The model under review builds one solid part; all positions refer to its coordinate system, in mm. A direction names the side the tool comes from. Round coordinates to 2 decimals unless told otherwise and drop trailing zeros. Order: outer loops, then holes, each group sorted by start corner. A loop starts at its lowest first (then second) coordinate and runs counter-clockwise, first axis right, second up. Notation, with made-up numbers: (8.25, 76.5) - (45.25, 76.5) arc R16 cw to (45.25, 95.5) - close; hole circle Ø1 at (-18.5, 79.5). An arc over 180 degrees is marked (long way). One line per question, with ' | ' between items. Start each with the question number.
Item 1: Add section B-B on x = 1. State the section outline as (y, z) points, and give its area (3 significant figures).
Item 2: Add section D-D on z = -12.5. State the section outline as (x, y) points.
Item 3: Insertion check: pin 1 Ø1 at (y, z) = (-30, 18.5) entering from +X; pin 2 Ø10 at (y, z) = (-12.5, -15.5) entering from +X; pin 3 Ø3 at (x, z) = (26, 17.32) entering from +Y; pin 4 Ø7.5 at (y, z) = (6.5, 4) entering from -X. Each pin has a flat end and moves straight along its axis. Give the tip position at first contact, or say it passes through.
Item 4: Tool access review of faces 1 (the face through (1, 0, 0)), 2 (the face through (-30, 6, -6)), 3 (the face through (27.476, -51.521, -18.261)), 4 (the face through (9, 6, 22)), 5 (the face through (-18, 7, -21)): name each direction out of +Z, -Z, +X, -X, +Y, -Y from which nothing blocks a thin tool from reaching the whole face with its end or side.
Item 5: For L1, parallel to X at y = -51, z = 0; L2, parallel to Y at x = -24, z = 4.5; L3, parallel to Z at x = -15, y = -23.5, list the stretches that pass through material, from the lowest coordinate up. Write a range as [from, to].
Item 6: Add section A-A on y = 6. State the section outline as (x, z) points, and give its area (3 significant figures).
Item 7: Draft analysis for pull direction X (two halves, no side actions). For faces 6 (the face through (-31, -21, 0)), 7 (the face through (-30, 6, 6)), 8 (the face through (-7, 6, -22)), state which applies: +X half, -X half, draft (parallel to the pull), parting line (faces both ways), or undercut.
Item 8: Add section C-C on x = -13.5. State the section outline as (y, z) points.
from build123d import *

# Parameters (mm, degrees)
SKETCH_1_W          = 62
SKETCH_1_H          = 46
EXTRUDE_1_DEPTH     = 10
SKETCH_2_W          = 58
SKETCH_2_H          = 42
CUT_EXTRUDE_1_DEPTH = 7
CUT_EXTRUDE_2_REACH = 68.88
SKETCH_3_W          = 12
SKETCH_3_H          = 14
CUT_EXTRUDE_3_REACH = 56.745
SKETCH_5_W          = 36
SKETCH_5_H          = 7
CUT_EXTRUDE_4_REACH = 56.745
SKETCH_6_W          = 20
SKETCH_6_H          = 7
EXTRUDE_2_DEPTH     = 50
SKETCH_9_W          = 62
SKETCH_9_H          = 46
EXTRUDE_3_DEPTH     = 3
CUT_EXTRUDE_5_REACH = 75.885
SKETCH_10_R         = 1.75


with BuildPart() as part:
    # 草图1 → 凸台-拉伸1 (new body)
    with BuildSketch(Plane(origin=(0, 0, 0), x_dir=(1, 0, 0), z_dir=(0, 1, 0))):
        Rectangle(SKETCH_1_W, SKETCH_1_H)
    extrude(amount=EXTRUDE_1_DEPTH)

    # 草图2 → 切除-拉伸1 (cut)
    with BuildSketch(Plane(origin=(0, 10, 0), x_dir=(1, 0, 0), z_dir=(0, 1, 0))):
        Rectangle(SKETCH_2_W, SKETCH_2_H)
    extrude(amount=-CUT_EXTRUDE_1_DEPTH, mode=Mode.SUBTRACT)

    # 草图3 → 切除-拉伸2 (cut, up to next)
    with BuildSketch(Plane.ZY.offset(31), mode=Mode.PRIVATE) as cut_extrude_2_sk1:
        with Locations((0, 10)):
            Rectangle(SKETCH_3_W, SKETCH_3_H)
    cut_extrude_2_tool1 = extrude(cut_extrude_2_sk1.sketch, amount=-CUT_EXTRUDE_2_REACH, mode=Mode.PRIVATE) & part.part
    add(cut_extrude_2_tool1.solids().sort_by_distance((-31, 10, 0))[0], mode=Mode.SUBTRACT)

    # 草图5 → 切除-拉伸3 (cut, up to next)
    with BuildSketch(Plane.XY.offset(-21), mode=Mode.PRIVATE) as cut_extrude_3_sk1:
        with Locations((11, 6.5)):
            Rectangle(SKETCH_5_W, SKETCH_5_H)
    cut_extrude_3_tool1 = extrude(cut_extrude_3_sk1.sketch, amount=-CUT_EXTRUDE_3_REACH, mode=Mode.PRIVATE) & part.part
    add(cut_extrude_3_tool1.solids().sort_by_distance((11, 6.5, -21))[0], mode=Mode.SUBTRACT)

    # 草图6 → 切除-拉伸4 (cut, up to next)
    with BuildSketch(Plane(origin=(0, 0, 21), x_dir=(-1, 0, 0), z_dir=(0, 0, -1)), mode=Mode.PRIVATE) as cut_extrude_4_sk1:
        with Locations((-19, 6.5)):
            Rectangle(SKETCH_6_W, SKETCH_6_H)
    cut_extrude_4_tool1 = extrude(cut_extrude_4_sk1.sketch, amount=-CUT_EXTRUDE_4_REACH, mode=Mode.PRIVATE) & part.part
    add(cut_extrude_4_tool1.solids().sort_by_distance((19, 6.5, 21))[0], mode=Mode.SUBTRACT)

    # 草图8 → 凸台-拉伸2 (add)
    with BuildSketch(Plane.XZ):
        Polygon((0, -23), (0, -20), (-28, -20), (-28, 20), (0, 20), (0, 23), (-31, 23), (-31, -23), align=None)
    extrude(amount=EXTRUDE_2_DEPTH)

    # 草图9 → 凸台-拉伸3 (add)
    with BuildSketch(Plane.XZ.offset(50)):
        Rectangle(SKETCH_9_W, SKETCH_9_H)
    extrude(amount=EXTRUDE_3_DEPTH)

    # 草图10 → 切除-拉伸5 (cut, up to next)
    with BuildSketch(Plane.XZ.offset(53), mode=Mode.PRIVATE) as cut_extrude_5_sk1:
        with BuildLine():
            Line((31, 17.435595774), (31, 23))
            Line((31, 23), (16, 23))
            ThreePointArc((16, 23), (23.999415516, 21.564075482), (31, 17.435595774))
        make_face()
    cut_extrude_5_tool1 = extrude(cut_extrude_5_sk1.sketch, amount=-CUT_EXTRUDE_5_REACH, mode=Mode.PRIVATE) & part.part
    # 草图10 → 切除-拉伸5 (cut, up to next)
    with BuildSketch(Plane.XZ.offset(53), mode=Mode.PRIVATE) as cut_extrude_5_sk2:
        with BuildLine():
            ThreePointArc((31, -17.435595774), (23.999415516, -21.564075482), (16, -23))
            Line((16, -23), (31, -23))
            Line((31, -23), (31, -17.435595774))
        make_face()
    cut_extrude_5_tool2 = extrude(cut_extrude_5_sk2.sketch, amount=-CUT_EXTRUDE_5_REACH, mode=Mode.PRIVATE) & part.part
    # 草图10 → 切除-拉伸5 (cut, up to next)
    with BuildSketch(Plane.XZ.offset(53), mode=Mode.PRIVATE) as cut_extrude_5_sk3:
        with Locations(Location((26, -17.320508076, 0), (0, 0, 270))):
            Circle(SKETCH_10_R)
    cut_extrude_5_tool3 = extrude(cut_extrude_5_sk3.sketch, amount=-CUT_EXTRUDE_5_REACH, mode=Mode.PRIVATE) & part.part
    # 草图10 → 切除-拉伸5 (cut, up to next)
    with BuildSketch(Plane.XZ.offset(53), mode=Mode.PRIVATE) as cut_extrude_5_sk4:
        with Locations(Location((26, 17.320508076, 0), (0, 0, 270))):
            Circle(SKETCH_10_R)
    cut_extrude_5_tool4 = extrude(cut_extrude_5_sk4.sketch, amount=-CUT_EXTRUDE_5_REACH, mode=Mode.PRIVATE) & part.part
    # 草图10 → 切除-拉伸5 (cut, up to next)
    with BuildSketch(Plane.XZ.offset(53), mode=Mode.PRIVATE) as cut_extrude_5_sk5:
        with BuildLine():
            ThreePointArc((27.5, 0), (24.131727984, 8.131727984), (16, 11.5))
            Line((16, 11.5), (16, -11.5))
            ThreePointArc((16, -11.5), (24.131727984, -8.131727984), (27.5, 0))
        make_face()
    cut_extrude_5_tool5 = extrude(cut_extrude_5_sk5.sketch, amount=-CUT_EXTRUDE_5_REACH, mode=Mode.PRIVATE) & part.part
    # 草图10 → 切除-拉伸5 (cut, up to next)
    with BuildSketch(Plane.XZ.offset(53), mode=Mode.PRIVATE) as cut_extrude_5_sk6:
        with BuildLine():
            Line((16, -11.5), (16, 11.5))
            ThreePointArc((16, 11.5), (4.5, 0), (16, -11.5))
        make_face()
    cut_extrude_5_tool6 = extrude(cut_extrude_5_sk6.sketch, amount=-CUT_EXTRUDE_5_REACH, mode=Mode.PRIVATE) & part.part
    # 草图10 → 切除-拉伸5 (cut, up to next)
    with BuildSketch(Plane.XZ.offset(53), mode=Mode.PRIVATE) as cut_extrude_5_sk7:
        with BuildLine():
            ThreePointArc((27.5, 0), (24.131727984, 8.131727984), (16, 11.5))
            Line((16, 11.5), (16, -11.5))
            ThreePointArc((16, -11.5), (24.131727984, -8.131727984), (27.5, 0))
        make_face()
    cut_extrude_5_tool7 = extrude(cut_extrude_5_sk7.sketch, amount=-CUT_EXTRUDE_5_REACH, mode=Mode.PRIVATE) & part.part
    # 草图10 → 切除-拉伸5 (cut, up to next)
    with BuildSketch(Plane.XZ.offset(53), mode=Mode.PRIVATE) as cut_extrude_5_sk8:
        with BuildLine():
            Line((16, -11.5), (16, 11.5))
            ThreePointArc((16, 11.5), (4.5, 0), (16, -11.5))
        make_face()
    cut_extrude_5_tool8 = extrude(cut_extrude_5_sk8.sketch, amount=-CUT_EXTRUDE_5_REACH, mode=Mode.PRIVATE) & part.part
    # 草图10 → 切除-拉伸5 (cut, up to next)
    with BuildSketch(Plane.XZ.offset(53), mode=Mode.PRIVATE) as cut_extrude_5_sk9:
        with Locations(Location((-4, 0, 0), (0, 0, 270))):
            Circle(SKETCH_10_R)
    cut_extrude_5_tool9 = extrude(cut_extrude_5_sk9.sketch, amount=-CUT_EXTRUDE_5_REACH, mode=Mode.PRIVATE) & part.part
    add(cut_extrude_5_tool1.solids().sort_by_distance((27.346788, -53, 21.372088))[0], mode=Mode.SUBTRACT)
    add(cut_extrude_5_tool2.solids().sort_by_distance((27.346788, -53, -21.372088))[0], mode=Mode.SUBTRACT)
    add(cut_extrude_5_tool3.solids().sort_by_distance((26, -53, -17.320508))[0], mode=Mode.SUBTRACT)
    add(cut_extrude_5_tool4.solids().sort_by_distance((26, -53, 17.320508))[0], mode=Mode.SUBTRACT)
    add(cut_extrude_5_tool5.solids().sort_by_distance((20.880752, -53, 0))[0], mode=Mode.SUBTRACT)
    add(cut_extrude_5_tool6.solids().sort_by_distance((11.119248, -53, 0))[0], mode=Mode.SUBTRACT)
    add(cut_extrude_5_tool7.solids().sort_by_distance((20.880752, -53, 0))[0], mode=Mode.SUBTRACT)
    add(cut_extrude_5_tool8.solids().sort_by_distance((11.119248, -53, 0))[0], mode=Mode.SUBTRACT)
    add(cut_extrude_5_tool9.solids().sort_by_distance((-4, -53, 0))[0], mode=Mode.SUBTRACT)


solid = part.part
Determined:
1) outline: (-53, -23) - (-50, -23) - (-50, 23) - (-53, 23) - close; (0, -23) - (3, -23) - (3, 21) - (10, 21) - (10, 23) - (0, 23) - close | area: 290 mm2
2) outline: (-31, -53) - (31, -53) - (31, -50) - (-28, -50) - (-28, 0) - (31, 0) - (31, 10) - (29, 10) - (29, 3) - (-29, 3) - (-29, 10) - (-31, 10) - close
3) pin 1: x = -28 | pin 2: x = 0 | pin 3: y = 3 | pin 4: x = -31
4) face 1: +X | face 2: -X, +Y | face 3: -Y | face 4: +Z, -Z, +Y | face 5: +Y
5) L1: [-31, -5.75], [-2.25, 4.5], [27.5, 31] | L2: [-53, -50], [0, 3] | L3: [-23, -20], [20, 23]
6) outline: (-31, -23) - (-7, -23) - (-7, -21) - (-29, -21) - (-29, -6) - (-31, -6) - close; (-31, 6) - (-29, 6) - (-29, 21) - (9, 21) - (9, 23) - (-31, 23) - close; (29, -23) - (31, -23) - (31, 23) - (29, 23) - close | area: 280 mm2
7) face 6: -X half | face 7: draft | face 8: undercut
8) outline: (-53, -23) - (10, -23) - (10, -21) - (3, -21) - (3, 21) - (10, 21) - (10, 23) - (-53, 23) - close; hole (-50, -20) - (0, -20) - (0, 20) - (-50, 20) - close
